For this review, use the dimensioned drawing (mm, ordinates from the lowest corner) and the shaded views. A direction names the side the tool comes from. Round coordinates to 2 decimals unless told otherwise and drop trailing zeros. Order: outer loops, then holes, each group sorted by start corner. A loop starts at its lowest first (then second) coordinate and runs counter-clockwise, first axis right, second up. Notation, with made-up numbers: (1, 57.5) - (31, 57.5) arc R10 ccw to (31, 74.5) - close; hole circle Ø5 at (-5, 82.25). An arc over 180 degrees is marked (long way). Write each question's results on one line, items separated by ' | '. Start each with the question number.
(1) Take a section at A-A, the plane y = 13.5. Give the boundary of the cut face in (x, z) (3 decimals).
(2) For L1, parallel to Y at x = 65, z = 14.5 (3 decimals); L2, parallel to Z at x = 20.5, y = 6.5; L3, parallel to X at y = 1.5, z = 100 (3 decimals), list the stretches that pass through material, from the lowest coordinate up. Write a range as from..to.
(3) Take a section at C-C, the plane z = 67. Give the boundary of the cut face in (x, y) (3 decimals), plus the area to 3 significant figures.
(4) Take a section at B-B, the plane x = 73. Give the boundary of the cut face in (y, z) (3 decimals).
(5) For the marked faces 1 and 2, list the 3-axis set-ups (+Z, -Z, +X, -X, +Y, -Y) from which the entire face can be reached by the end or side of a thin tool; tool diameter is ignored.
(6) Take a section at D-D, the plane y = 1.5. Give the boundary of the cut face in (x, z) (3 decimals), plus the area to 3 significant figures.
(7) Insertion check: pin 1 Ø7 at (x, y) = (30.5, 13) entering from +Z (3 decimals); pin 2 Ø5 at (y, z) = (6, 47) entering from -X (3 decimals); pin 3 Ø6 at (x, z) = (91, 76.5) entering from -Y (3 decimals). Each pin has a flat end and moves straight along its axis. Give the tip position at first contact, or say it passes through.
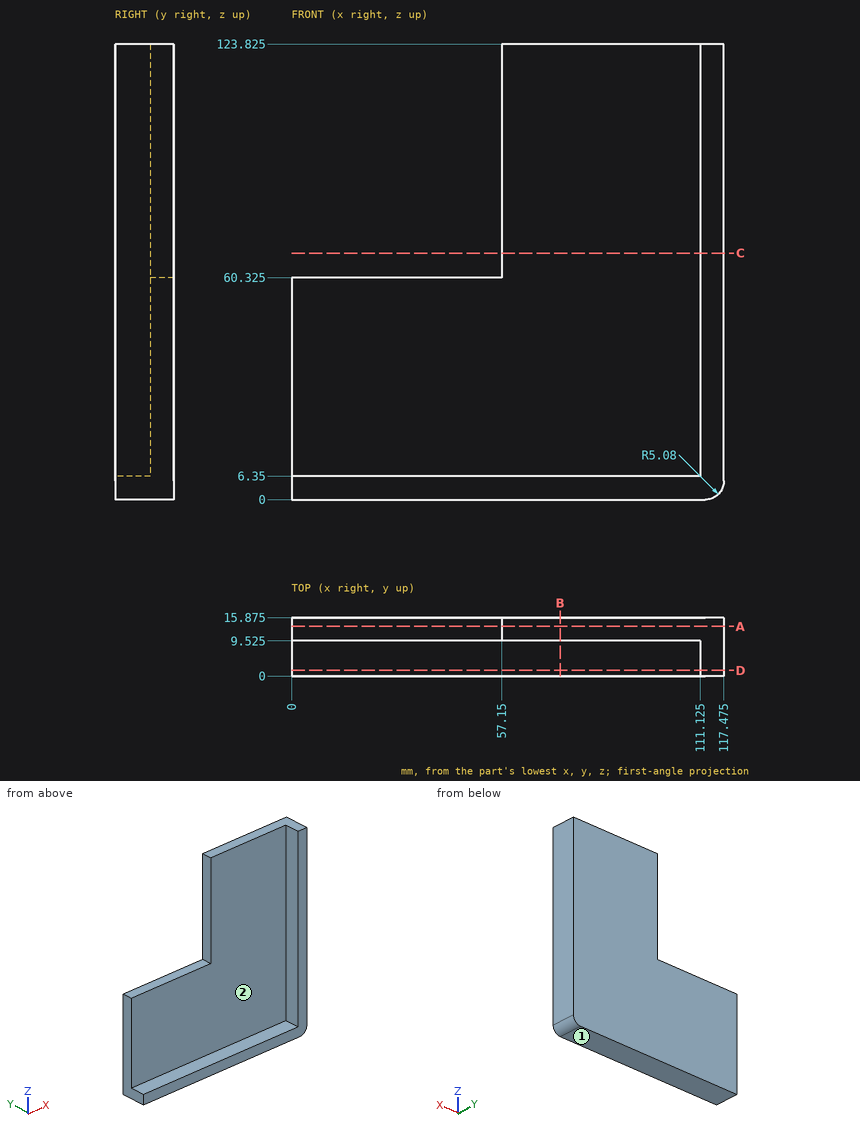
Results below:
1) outline: (0, 0) - (112.395, 0) arc R5.08 ccw to (117.475, 5.08) - (117.475, 123.825) - (57.15, 123.825) - (57.15, 60.325) - (0, 60.325) - close
2) L1: y = 9.525..15.875 | L2: z = 0..6.35 | L3: x = 111.125..117.475
3) outline: (57.15, 9.525) - (111.125, 9.525) - (111.125, 0) - (117.475, 0) - (117.475, 15.875) - (57.15, 15.875) - close | area: 444 mm^2
4) outline: (0, 0) - (15.875, 0) - (15.875, 123.825) - (9.525, 123.825) - (9.525, 6.35) - (0, 6.35) - close
5) face 1: -Z, +X, -X, +Y, -Y | face 2: +Z, -X, -Y
6) outline: (0, 0) - (112.395, 0) arc R5.08 ccw to (117.475, 5.08) - (117.475, 123.825) - (111.125, 123.825) - (111.125, 6.35) - (0, 6.35) - close | area: 1,490 mm^2
7) pin 1: stops at z = 60.325 | pin 2: stops at x = 111.125 | pin 3: stops at y = 9.525
